Here's how the part is built. I have some questions about the finished solid (model axes, mm). Face numbers are marked on the shaded views. A direction names the side the tool comes from. Round coordinates to 2 decimals unless told otherwise and drop trailing zeros. Order: outer loops, then holes, each group sorted by start corner. A loop starts at its lowest first (then second) coordinate and runs counter-clockwise, first axis right, second up. Notation, with made-up numbers: (1, 31.25) - (42, 31.25) arc R12 cw to (42, 41.25) - close; hole circle Ø10 at (73.5, 6). An arc over 180 degrees is marked (long way). Answer as a JSON object with one key per item and string values.
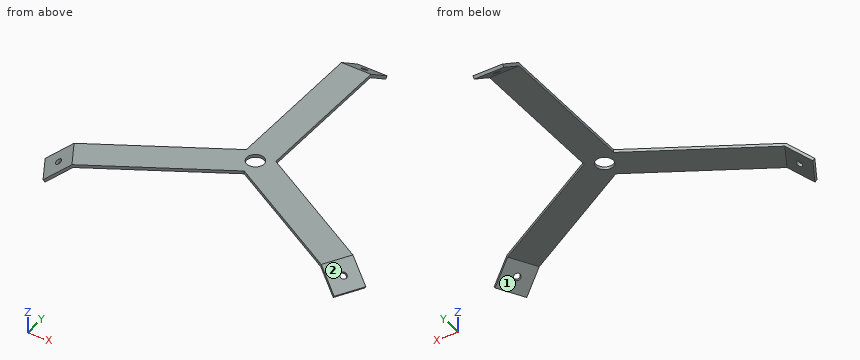
```python
from build123d import *

# Parameters (mm, degrees)
EXTRUDE_1_DEPTH          = 15
PATTERN_CIRCULAR_1_COUNT = 3
HOLE_WIZARD_M161_D       = 17.5
HOLE_WIZARD_M62_D        = 6.6
PATTERN_CIRCULAR_2_COUNT = 3


with BuildPart() as part:
    # Sketch 1 → Extrude 1 (new, symmetric)
    with BuildSketch(Plane(origin=(0, 0, 0), x_dir=(0, 0, -1), z_dir=(1, 0, 0))):
        Polygon((0, 0), (0, 155), (17.207293091, 179.574561329), (19.664749223, 177.85383202), (3, 154.054103633), (3, 0), align=None)
    extrude_1 = extrude(amount=EXTRUDE_1_DEPTH, both=True)

    # Pattern Circular 1: Extrude 1 ×3 about axis
    pattern_circular_1_axis = Axis((0, 0, 0), (0, 0, 1))
    for i in range(1, PATTERN_CIRCULAR_1_COUNT):
        add(extrude_1.rotate(pattern_circular_1_axis, i * 360 / PATTERN_CIRCULAR_1_COUNT))

    # Hole Wizard M161 (through all)
    with Locations(Plane(origin=(0, 0, -3), x_dir=(-1, 0, 0), z_dir=(0, 0, -1))):
        with Locations((0, 0)):
            Hole(HOLE_WIZARD_M161_D / 2)

    # Hole Wizard M62 (through all)
    with Locations(Plane(origin=(0, 165.566551355, -11.061102678), x_dir=(0, -0.819152044289, 0.573576436351), z_dir=(0, -0.573576436351, -0.819152044289))):
        with Locations((0, 0)):
            hole_wizard_m62 = Hole(HOLE_WIZARD_M62_D / 2)

    # Pattern Circular 2: Hole Wizard M62 ×3 about axis
    pattern_circular_2_axis = Axis((0, 0, 0), (0, 0, -1))
    for i in range(1, PATTERN_CIRCULAR_2_COUNT):
        add(hole_wizard_m62.rotate(pattern_circular_2_axis, i * 360 / PATTERN_CIRCULAR_2_COUNT), mode=Mode.SUBTRACT)


solid = part.part
```
1. Imagine slicing it at A-A (y = 0). List the corners of the cut face in (x, z) for me.
Responses:
{"outline": "(-30, -3) - (-8.75, -3) - (-8.75, 0) - (-30, 0) - close; (8.75, -3) - (30, -3) - (30, 0) - (8.75, 0) - close"}
2. For the marked faces 1 and 2, which set-ups out of +Z, -Z, +X, -X, +Y, -Y let a thin tool reach every point of the face, with its end or its side?
Responses:
{"face 1": "-Z, +Y", "face 2": "+Z, +X, -Y"}
3. For P1, Ø10, axis at y = 83, z = -7, coming from the +X side; P2, Ø5, axis at x = 51, z = -7.5, coming from the -Y side; P3, Ø4, axis at y = -71.5, z = -4.5, coming from the +X side, each with a flat end and sliding along its axis, tell me the tip position at first contact or that it passes through.
Responses:
{"P1": "x = 15", "P2": "through", "P3": "x = 148.61"}
4. Imagine slicing it at B-B (x = 136). List the corners of the cut face in (y, z) for me, plus the area to 3 significant figures.
Responses:
{"outline": "(-95.84, -11.15) - (-72.55, -3) - (-61.2, -3) - (-61.2, 0) - (-74.44, 0) - (-95.84, -7.49) - close", "area": "119 mm2"}
5. If I drill on L1, parallel to Z at x = -3, y = 144; L2, parallel to Y at x = 0, z = -2.05; L3, parallel to X at y = 92.5, z = -2.75, over which ranges is the centre line in solid material (lowest first)? Write a range as [from, to].
Responses:
{"L1": "[-3, 0]", "L2": "[-17.32, -8.75], [8.75, 157.93]", "L3": "[-15, 15]"}
6. Imagine slicing it at C-C (x = 55). List the corners of the cut face in (y, z) for me, plus the area to 3 significant figures.
Responses:
{"outline": "(-49.07, -3) - (-14.43, -3) - (-14.43, 0) - (-49.07, 0) - close", "area": "104 mm2"}
